Could you check a few things on this model? Use its own coordinates, in mm. Face numbers are marked on the shaded views. Coordinates: 2 decimals unless noted, no trailing zeros. Loops run counter-clockwise (first coordinate to the right, second up) from the corner with the lowest first, then second, coordinate; pieces in that order, holes last.
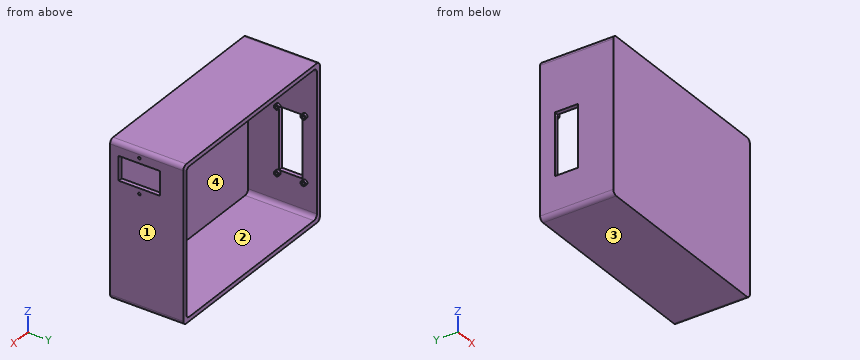
from build123d import *

# Parameters (mm, degrees)
SKETCH1_W           = 230
SKETCH1_H           = 180
BOSS_EXTRUDE1_DEPTH = 5
SKETCH2_W           = 230
SKETCH2_H           = 180
SKETCH2_W_2         = 220
SKETCH2_H_2         = 170
BOSS_EXTRUDE2_DEPTH = 80
FILLET1_R           = 5
SKETCH3_W           = 28
SKETCH3_H           = 48
CUT_EXTRUDE1_DEPTH  = 5
SKETCH4_R           = 1.5
CUT_EXTRUDE2_DEPTH  = 5
SKETCH7_R           = 3
BOSS_EXTRUDE3_DEPTH = 3
SKETCH5_W           = 72
SKETCH5_H           = 27
CUT_EXTRUDE3_DEPTH  = 10
SKETCH8_R           = 1.5
CUT_EXTRUDE4_DEPTH  = 5


with BuildPart() as part:
    # Sketch1 → Boss-Extrude1 (new body)
    with BuildSketch(Plane(origin=(0, 0, 0), x_dir=(1, 0, 0), z_dir=(0, 1, 0))):
        with Locations((115, 90)):
            Rectangle(SKETCH1_W, SKETCH1_H)
    extrude(amount=BOSS_EXTRUDE1_DEPTH)

    # Sketch2 → Boss-Extrude2 (add)
    with BuildSketch(Plane(origin=(0, 5, 0), x_dir=(1, 0, 0), z_dir=(0, 1, 0))):
        with Locations((115, 90)):
            Rectangle(SKETCH2_W, SKETCH2_H)
        with Locations((115, 90)):
            Rectangle(SKETCH2_W_2, SKETCH2_H_2, mode=Mode.SUBTRACT)
    extrude(amount=BOSS_EXTRUDE2_DEPTH)

    # Fillet1
    fillet1_edges = [part.edges().sort_by_distance(p)[0] for p in [
        (225, 45, -5),
        (225, 45, -175),
        (5, 45, -175),
        (5, 45, -5),
        (0, 42.5, -180),
        (230, 42.5, -180),
        (230, 42.5, 0),
        (0, 42.5, 0),
    ]]
    fillet(fillet1_edges, radius=FILLET1_R)

    # Sketch3 → Cut-Extrude1 (cut)
    with BuildSketch(Plane(origin=(230, 0, 0), x_dir=(0, 0, -1), z_dir=(1, 0, 0))):
        with Locations((29, 34)):
            Rectangle(SKETCH3_W, SKETCH3_H)
    extrude(amount=-CUT_EXTRUDE1_DEPTH, mode=Mode.SUBTRACT)

    # Sketch4 → Cut-Extrude2 (cut)
    with BuildSketch(Plane(origin=(230, 0, 0), x_dir=(0, 0, -1), z_dir=(1, 0, 0))):
        with Locations((9, 34)):
            Circle(SKETCH4_R)
        with Locations((49.4, 34)):
            Circle(SKETCH4_R)
    extrude(amount=-CUT_EXTRUDE2_DEPTH, mode=Mode.SUBTRACT)

    # Sketch7 → Boss-Extrude3 (add)
    with BuildSketch(Plane(origin=(5, 0, 0), x_dir=(0, 0, -1), z_dir=(1, 0, 0))):
        with Locations((139, 40)):
            Circle(SKETCH7_R)
        with Locations((139, 71)):
            Circle(SKETCH7_R)
        with Locations((64, 71)):
            Circle(SKETCH7_R)
        with Locations((64, 40)):
            Circle(SKETCH7_R)
    extrude(amount=BOSS_EXTRUDE3_DEPTH)

    # Sketch5 → Cut-Extrude3 (cut)
    with BuildSketch(Plane.ZY):
        with Locations((-100, 54.5)):
            Rectangle(SKETCH5_W, SKETCH5_H)
    extrude(amount=-CUT_EXTRUDE3_DEPTH, mode=Mode.SUBTRACT)

    # Sketch8 → Cut-Extrude4 (cut)
    with BuildSketch(Plane(origin=(8, 0, 0), x_dir=(0, 0, -1), z_dir=(1, 0, 0))):
        with Locations((64, 40)):
            Circle(SKETCH8_R)
        with Locations((139, 40)):
            Circle(SKETCH8_R)
        with Locations((139, 71)):
            Circle(SKETCH8_R)
        with Locations((64, 71)):
            Circle(SKETCH8_R)
    extrude(amount=-CUT_EXTRUDE4_DEPTH, mode=Mode.SUBTRACT)


solid = part.part
1) Imagine slicing it at C-C on y = 19. List the corners of the cut face in (x, z) for me.
2) Imagine slicing it at A-A on z = -102.5. List the corners of the cut face in (x, y) for me.
3) Imagine slicing it at D-D on x = 23.5. List the corners of the cut face in (y, z) for me.
4) Imagine slicing it at B-B on y = 49.5. List the corners of the cut face in (x, z) for me.
5) We'd pull the mould along Z, two halves only. Please class the marked faces 1, 2, 3 and 4: released by +Z, released by -Z, zero draft, split by the parting line, or undercut.
6) If I drill on L1, parallel to Z at x = 4.8, y = 71; L2, parallel to Y at x = 226.3, z = -49.4; L3, parallel to Z at x = 136.5, y = 14.5, over which ranges is the centre line in solid material (lowest first)?
7) Will these pins go through, and if not, where does the flat tip stop? pin 1 (5.5 mm diameter, centred on x = 228, y = 28, fed in from -Z); pin 2 (2 mm diameter, centred on x = 199.5, z = -86.5, fed in from +Y); pin 3 (4 mm diameter, centred on x = 228.5, y = 24, fed in from +Z).
Solved:
1. outline: (0, -175) arc R5 ccw to (5, -180) - (225, -180) arc R5 ccw to (230, -175) - (230, -43) - (225, -43) - (225, -170) arc R5 cw to (220, -175) - (10, -175) arc R5 cw to (5, -170) - (5, -10) arc R5 cw to (10, -5) - (220, -5) arc R5 cw to (225, -10) - (225, -15) - (230, -15) - (230, -5) arc R5 ccw to (225, 0) - (5, 0) arc R5 ccw to (0, -5) - close
2. outline: (0, 0) - (230, 0) - (230, 85) - (225, 85) - (225, 5) - (5, 5) - (5, 41) - (0, 41) - close; (0, 68) - (5, 68) - (5, 85) - (0, 85) - close
3. outline: (0, -180) - (85, -180) - (85, -175) - (5, -175) - (5, -5) - (85, -5) - (85, 0) - (0, 0) - close
4. outline: (0, -175) arc R5 ccw to (5, -180) - (225, -180) arc R5 ccw to (230, -175) - (230, -43) - (225, -43) - (225, -170) arc R5 cw to (220, -175) - (10, -175) arc R5 cw to (5, -170) - (5, -136) - (0, -136) - close; (0, -64) - (5, -64) - (5, -10) arc R5 cw to (10, -5) - (220, -5) arc R5 cw to (225, -10) - (225, -15) - (230, -15) - (230, -5) arc R5 ccw to (225, 0) - (5, 0) arc R5 ccw to (0, -5) - close
5. face 1: zero draft
5. face 2: undercut
5. face 3: released by -Z
5. face 4: undercut
6. L1: z = -180 to -140.5, -137.5 to -65.5, -62.5 to 0
6. L2: y = 0 to 32.5, 35.5 to 85
6. L3: z = -180 to -175, -5 to 0
7. pin 1: stops at z = -179.99
7. pin 2: stops at y = 5
7. pin 3: stops at z = -0.23
